Work out the finished part from the listing and answer in its coordinate system (mm). Round coordinates to 2 decimals unless told otherwise and drop trailing zeros. Order: outer loops, then holes, each group sorted by start corner. A loop starts at its lowest first (then second) coordinate and runs counter-clockwise, first axis right, second up. Notation, with made-up numbers: M -11.5,74.25 L 38.5,74.25 A21 cw 38.5,95.25 Z; hole C 24,-12 d9. An arc over 180 degrees is marked long. Return JSON: item names as keys, results as strings.
Solid Edge part; units mm, degrees
sketch "Sketch1" plane through (0, 0, 0) normal (1, 0, 0) x (0, 1, 0)
  line L0 (27.5, -27) -> (27.5, 23)
  line L1 (27.5, 23) -> (-31.5, 23)
  line L2 (-31.5, 23) -> (-31.5, -27)
  line L3 (-31.5, -27) -> (27.5, -27)
extrude "Protrusion1" add sketch "Sketch1" along normal blind 2
sketch "Sketch2" plane through (0, 0, 0) normal (1, 0, 0) x (0, 1, 0)
  line L0 (-31.5, 21) -> (-7, 21)
  line L1 (-7, 21) -> (-7, 23)
  line L2 (-7, 23) -> (-31.5, 23)
  line L3 (-31.5, 23) -> (-31.5, 21)
extrude "ExtrudedCutout_1" cut sketch "Sketch2" along normal blind 2
sketch "Sketch3" plane through (0, 0, 0) normal (1, 0, 0) x (0, 1, 0)
  line L0 (3, 21) -> (27.5, 21)
  line L1 (27.5, 21) -> (27.5, 23)
  line L2 (27.5, 23) -> (3, 23)
  line L3 (3, 23) -> (3, 21)
extrude "ExtrudedCutout_2" cut sketch "Sketch3" along normal blind 2
sketch "Sketch4" plane through (0, 0, 0) normal (1, 0, 0) x (0, 1, 0)
  line L0 (23.5, 3) -> (23.5, -7)
  line L1 (23.5, -7) -> (25.5, -7)
  line L2 (25.5, -7) -> (25.5, 3)
  line L3 (25.5, 3) -> (23.5, 3)
extrude "ExtrudedCutout_3" cut sketch "Sketch4" along normal blind 2
sketch "Sketch5" plane through (0, 0, 0) normal (1, 0, 0) x (0, 1, 0)
  line L0 (27.5, -25) -> (3, -25)
  line L1 (3, -25) -> (3, -27)
  line L2 (3, -27) -> (27.5, -27)
  line L3 (27.5, -27) -> (27.5, -25)
extrude "ExtrudedCutout_4" cut sketch "Sketch5" along normal blind 4
sketch "Sketch6" plane through (0, 0, 0) normal (1, 0, 0) x (0, 1, 0)
  line L0 (-7, -25) -> (-31.5, -25)
  line L1 (-31.5, -25) -> (-31.5, -27)
  line L2 (-31.5, -27) -> (-7, -27)
  line L3 (-7, -27) -> (-7, -25)
extrude "ExtrudedCutout_5" cut sketch "Sketch6" along normal blind 2
sketch "Sketch7" plane through (0, 0, 0) normal (1, 0, 0) x (0, 1, 0)
  line L0 (-29.5, -7) -> (-27.5, -7)
  line L1 (-27.5, -7) -> (-27.5, 3)
  line L2 (-27.5, 3) -> (-29.5, 3)
  line L3 (-29.5, 3) -> (-29.5, -7)
extrude "ExtrudedCutout_6" cut sketch "Sketch7" along normal blind 4
sketch "Sketch8" plane through (0, 0, 0) normal (1, 0, 0) x (0, 1, 0)
  line L0 (8, 8) -> (-10.5, 8)
  line L1 (-10.5, 8) -> (-10.5, -2)
  line L2 (-10.5, -2) -> (8, -2)
  line L3 (8, -2) -> (8, 8)
  circle A0 centre (-13.745, 3) radius 1.98
  circle A1 centre (11.245, 3) radius 1.98
extrude "ExtrudedCutout_9" cut sketch "Sketch8" along normal blind 2
sketch "Sketch9" plane through (0, 0, 0) normal (1, 0, 0) x (0, 1, 0)
  circle A0 centre (-2.5, -12.5) radius 3
extrude "ExtrudedCutout_10" cut sketch "Sketch9" along normal blind 2
fillet "Round_1" radius 1 4 edges at (1, 27.5, -25) (1, 27.5, 21) (1, -31.5, -25) (1, -31.5, 21)
properties material "Acrylic, high impact grade"
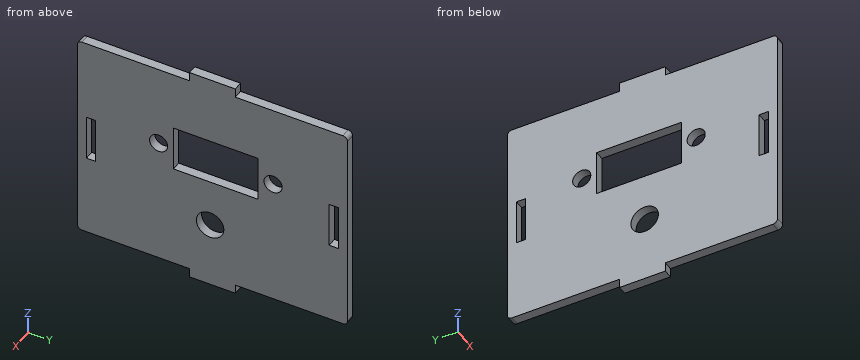
Item 1: Find section A-A (z = 0). Determine the outline of the cut face in (x, y), plus the area to 3 significant figures.
Output:
{"outline": "M 0,-31.5 L 2,-31.5 L 2,-29.5 L 0,-29.5 Z; M 0,-27.5 L 2,-27.5 L 2,-10.5 L 0,-10.5 Z; M 0,8 L 2,8 L 2,23.5 L 0,23.5 Z; M 0,25.5 L 2,25.5 L 2,27.5 L 0,27.5 Z", "area": "73.0 mm^2"}
Item 2: Each of these flat-tipped pins is pushed along its axis until it touches: pin 1 (0.6 mm diameter, centred on x = 1, z = 22, fed in from +Y); pin 2 (0.6 mm diameter, centred on x = 1, z = 21.5, fed in from -Y); pin 3 (1 mm diameter, centred on x = 1, y = -21, fed in from +Z). Where does it stop, or does it pass through?
Output:
{"pin 1": "stops at y = 3", "pin 2": "stops at y = -7", "pin 3": "stops at z = 21"}
Item 3: Find section B-B (x = 1.15). State how many separate pieces and enclosed holes the cut face has, plus the area to 3 significant figures.
Output:
{"separate pieces": "1", "enclosed holes": "6", "area": "2,480 mm^2"}
Item 4: Find section C-C (z = -12.5). Determine the outline of the cut face in (x, y), plus the area to 3 significant figures.
Output:
{"outline": "M 0,-31.5 L 2,-31.5 L 2,-5.5 L 0,-5.5 Z; M 0,0.5 L 2,0.5 L 2,27.5 L 0,27.5 Z", "area": "106 mm^2"}
Item 5: Consider line 1 along Z through (x, y) = (1.45, -2.5); line 2 along Y through (x, z) = (1.5, 0); line 3 along Y through (x, z) = (1.4, 4.5). Determine where each line is inside the solid, lowest interval first. Write a range as [from, to].
Output:
{"line 1": "z = [-27, -15.5], [-9.5, -2], [8, 23]", "line 2": "y = [-31.5, -29.5], [-27.5, -10.5], [8, 23.5], [25.5, 27.5]", "line 3": "y = [-31.5, -15.04], [-12.45, -10.5], [8, 9.95], [12.54, 27.5]"}
Item 6: Find section D-D (y = -2.5). Determine the outline of the cut face in (x, z), plus the area to 3 significant figures.
Output:
{"outline": "M 0,-27 L 2,-27 L 2,-15.5 L 0,-15.5 Z; M 0,-9.5 L 2,-9.5 L 2,-2 L 0,-2 Z; M 0,8 L 2,8 L 2,23 L 0,23 Z", "area": "68.0 mm^2"}
